Verification items for the finished model (mm, model axes). Face numbers are marked on the shaded views. A direction names the side the tool comes from. Coordinates: 2 decimals unless noted, no trailing zeros. Loops run counter-clockwise (first coordinate to the right, second up) from the corner with the lowest first, then second, coordinate; pieces in that order, holes last. Notation, with made-up numbers: (-38, -35) - (13, -35) arc R17 cw to (13, -23) - close; hole circle Ø6 at (67, 86). An arc over 180 degrees is marked (long way). One line per item, written item: value. Start each with the question number.
(1) Section check C-C (z = 37). Record the boundary of the cut face in (x, y).
(2) Gauge pin test, flat ends, axial feed: P1, Ø20, axis at x = 33.5, y = 36, coming from the +Z side; P2, Ø3, axis at x = 28.5, z = 26, coming from the +Y side; P3, Ø7.5, axis at y = 53, z = -29.5, coming from the +X side. Record the tip position at first contact, or that the pin passes through.
(3) Draft check along X on the marked faces 4, 5 and 6. Enter one of: +X half, -X half, draft (parallel to the pull), parting line (faces both ways), or undercut.
(4) Set-up check for the marked faces 1, 2 and 3: record each of +Z, -Z, +X, -X, +Y, -Y from which the full face is reachable in a straight line by a thin tool's end or side.
(5) Section check B-B (x = 16). Record the boundary of the cut face in (y, z), plus the area to 3 significant figures.
(6) Section check A-A (y = 15). Record the boundary of the cut face in (x, z).
(7) Thickness scan on probe 1 along Z at (x, y) = (33, 14.5); probe 2 along X at (y, z) = (35.5, 24); probe 3 along Y at (x, z) = (18, -25). Record the ranges inside material, lowest first. Write a range as [from, to].
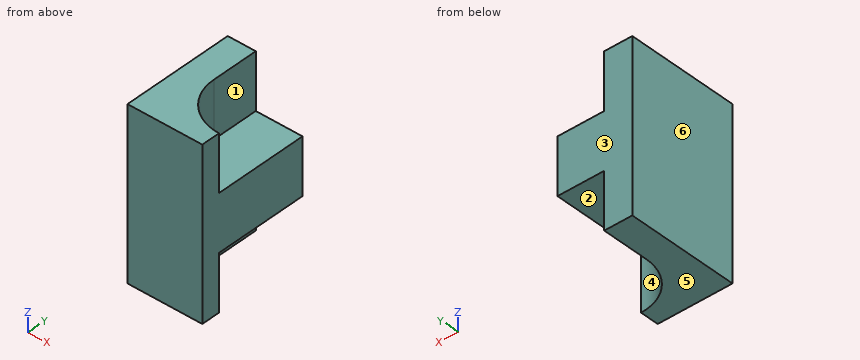
```python
from build123d import *

# Parameters (mm, degrees)
BOSS_EXTRUDE1_DEPTH = 45
BOSS_EXTRUDE2_DEPTH = 15


with BuildPart() as part:
    # Sketch1 → Boss-Extrude1 (new, symmetric)
    with BuildSketch(Plane.XY):
        with BuildLine():
            Line((0, 0), (40, 0))
            Line((40, 0), (40, 10))
            ThreePointArc((40, 10), (22.32233047, 17.32233047), (15, 35))
            Line((15, 35), (15, 60))
            Line((15, 60), (0, 60))
            Line((0, 60), (0, 0))
        make_face()
    extrude(amount=BOSS_EXTRUDE1_DEPTH, both=True)

    # Sketch1<3> → Boss-Extrude2 (add, symmetric)
    with BuildSketch(Plane.XY):
        with BuildLine():
            ThreePointArc((15, 35), (22.32233047, 17.32233047), (40, 10))
            Line((40, 10), (40, 60))
            Line((40, 60), (15, 60))
            Line((15, 60), (15, 35))
        make_face()
    extrude(amount=BOSS_EXTRUDE2_DEPTH, both=True)


solid = part.part
```
Responses:
1. outline: (0, 0) - (40, 0) - (40, 10) arc R25 cw to (15, 35) - (15, 60) - (0, 60) - close
2. P1: stops at z = 15
2. P2: stops at y = 13.65
2. P3: stops at x = 15
3. face 4: +X half
3. face 5: draft
3. face 6: -X half
4. face 1: +Z, +X, +Y
4. face 2: -Z, +X, +Y
4. face 3: +Z, -Z, +X, -X, +Y
5. outline: (0, -45) - (28, -45) - (28, -15) - (60, -15) - (60, 15) - (28, 15) - (28, 45) - (0, 45) - close
5. area: 3,480 mm²
6. outline: (0, -45) - (25, -45) - (25, -15) - (40, -15) - (40, 15) - (25, 15) - (25, 45) - (0, 45) - close
7. probe 1: z = [-15, 15]
7. probe 2: x = [0, 15]
7. probe 3: y = [0, 23.13]
